```python
from build123d import *

# Parameters (mm, degrees)
SKETCH1_W           = 31
SKETCH1_H           = 14.3
BOSS_EXTRUDE1_DEPTH = 1.5
BOSS_EXTRUDE2_DEPTH = 14.3
SKETCH5_R           = 1.5
CUT_EXTRUDE1_DEPTH  = 1.5


with BuildPart() as part:
    # Sketch1 → Boss-Extrude1 (new body)
    with BuildSketch(Plane.XY):
        with Locations((15.5, 0)):
            Rectangle(SKETCH1_W, SKETCH1_H)
    extrude(amount=BOSS_EXTRUDE1_DEPTH)

    # Sketch2 → Boss-Extrude2 (add, through all)
    with BuildSketch(Plane.XZ.offset(7.15)):
        Polygon((2.5, 1.5), (2.5, 3.5), (0, 3.5), (0, 3), (2, 3), (2, 1.5), align=None)
    extrude(amount=-BOSS_EXTRUDE2_DEPTH)

    # Sketch4 → Revolve1 (revolve)
    with BuildSketch(Plane.XZ.offset(3.15)):
        with BuildLine():
            Line((0, 3.5), (0, 6))
            Line((0, 6), (-1, 6))
            Line((-1, 6), (-1, 5.65))
            Line((-1, 5.65), (-6.4, 5.65))
            ThreePointArc((-6.4, 5.65), (-8.097056275, 4.947056275), (-8.8, 3.25))
            Line((-8.8, 3.25), (0, 3.25))
            Line((0, 3.25), (0, 3.5))
        make_face()
    revolve1 = revolve(axis=Axis((0, -3.15, 3.25), (-1, 0, 0)))

    # Mirror1: Revolve1 across plane
    add(revolve1.mirror(Plane.ZX))

    # Sketch5 → Cut-Extrude1 (cut)
    with BuildSketch(Plane.XY.offset(1.5)):
        with Locations((25.5, 0)):
            Circle(SKETCH5_R)
    extrude(amount=-CUT_EXTRUDE1_DEPTH, mode=Mode.SUBTRACT)


solid = part.part
```
Source: CAD feature listing. Evaluate the final solid. Frame: model axes, mm. A direction names the side the tool comes from. Give positions to 0.01 mm unless a question says otherwise; leave off trailing zeros. Write each loop counter-clockwise with the first axis right and the second up, starting at its lowest first coordinate (ties: lowest second). Pieces come first, ordered by that corner, then holes.
1. Section query D-D (z = 4.7). Return the cut outline in (x, y).
2. First-contact query: pin 1 (4.5 mm diameter, centred on x = 18.5, y = 1.5, fed in from +Z); pin 2 (2 mm diameter, centred on x = 1.5, y = 0, fed in from +Z); pin 3 (1.2 mm diameter, centred on y = -3, z = 4.5, fed in from +X); pin 4 (2.5 mm diameter, centred on x = 25.5, y = 0, fed in from +Z). Flat tips, straight axial feed; report the tip coordinate or a pass-through.
3. Section query A-A (y = 0). Return the cut outline in (x, z), then the cut area to 3 significant figures.
4. Section query C-C (y = -3.15). Return the cut outline in (x, z).
5. Pull-direction query (Y, two-part tool) for faces 1 (the face through (15, -7.15, 1)), 2 (the face through (24, 0, 1)), 3 (the face through (15, 0, 0)); classes: +Y half, -Y half, draft (parallel to the pull), parting line (faces both ways), or undercut.
6. Material intervals for line 1 along Y through (x, z) = (-4, 3.3); line 2 along Y through (x, z) = (25.5, 0.7); line 3 along Z through (x, y) = (7, 4), sorted ascending.
7. Access query for faces 4 (the face through (0, 0, 1)), 5 (the face through (-0.507, -3.029, 0.503)), 6 (the face through (1, 0, 3)). Directions: +Z, -Z, +X, -X, +Y, -Y. A direction counts if a zero-diameter tool reaches every point of the face in a straight line with its end or side. Return the directions, or none.
8. Section query B-B (x = 25.5). Return the cut outline in (y, z), then the cut area to 4 significant figures.
Output values:
1. outline: (-6.4, -5.06) - (-1, -5.06) - (-1, -5.49) - (0, -5.49) - (0, -0.81) - (-1, -0.81) - (-1, -1.24) - (-6.4, -1.24) arc R1.91 ccw to start; (-6.4, 1.24) - (-1, 1.24) - (-1, 0.81) - (0, 0.81) - (0, 5.49) - (-1, 5.49) - (-1, 5.06) - (-6.4, 5.06) arc R1.91 ccw to start
2. pin 1: stops at z = 1.5
2. pin 2: stops at z = 3.5
2. pin 3: stops at x = 0
2. pin 4: passes through
3. outline: (0, 0) - (24, 0) - (24, 1.5) - (2.5, 1.5) - (2.5, 3.5) - (0, 3.5) - (0, 3) - (2, 3) - (2, 1.5) - (0, 1.5) - close; (27, 0) - (31, 0) - (31, 1.5) - (27, 1.5) - close
3. area: 44.0 mm2
4. outline: (-6.4, 0.85) - (-1, 0.85) - (-1, 0.5) - (0, 0.5) - (0, 0) - (31, 0) - (31, 1.5) - (2.5, 1.5) - (2.5, 3.5) - (0, 3.5) - (0, 6) - (-1, 6) - (-1, 5.65) - (-6.4, 5.65) arc R2.4 ccw to start; hole (0, 1.5) - (2, 1.5) - (2, 3) - (0, 3) - close
5. face 1: -Y half
5. face 2: undercut
5. face 3: draft
6. line 1: y = -5.55 to -0.75, 0.75 to 5.55
6. line 2: y = -7.15 to -1.5, 1.5 to 7.15
6. line 3: z = 0 to 1.5
7. face 4: -Z, -X
7. face 5: -X
7. face 6: +Y, -Y
8. outline: (-7.15, 0) - (-1.5, 0) - (-1.5, 1.5) - (-7.15, 1.5) - close; (1.5, 0) - (7.15, 0) - (7.15, 1.5) - (1.5, 1.5) - close
8. area: 16.95 mm2
